Here's the drawing with two shaded views (mm, measured from the low corner). I have some questions. Coordinates: 2 decimals unless noted, no trailing zeros. Order: outer loops, then holes, each group sorted by start corner. A loop starts at its lowest first (then second) coordinate and runs counter-clockwise, first axis right, second up. Notation, with made-up numbers: (62, -34.75) -> (66, -34.75) arc R36 ccw to (66, 3.25) -> close; hole circle Ø6 at (-31, 24). An arc over 180 degrees is marked (long way). Answer in a Markdown table with one row per item. Add a question column.
1. If I drill on line 1 along X through (y, z) = (2.9, 30); line 2 along Y through (x, z) = (7.5, 27); line 3 along Z through (x, y) = (18, 4.2), over which ranges is the centre line in solid material (lowest first)? Write a range as [from, to].
2. Imagine slicing it at A-A on x = 16. Write out the boundary of the cut face in (y, z).
3. Imagine slicing it at D-D on x = 50.5. Write out the boundary of the cut face in (y, z).
4. Imagine slicing it at C-C on y = 2.7. Write out the boundary of the cut face in (x, z), plus the area to 3 significant figures.
5. Imagine slicing it at B-B on z = 25. Write out the boundary of the cut face in (x, y), plus the area to 3 significant figures.
6. Will these pins go through, and if not, where does the flat tip stop? pin 1 (1.5 mm diameter, centred on x = 22.5, y = 3, fed in from +Z); pin 2 (1.5 mm diameter, centred on y = 3, z = 16.5, fed in from +X).
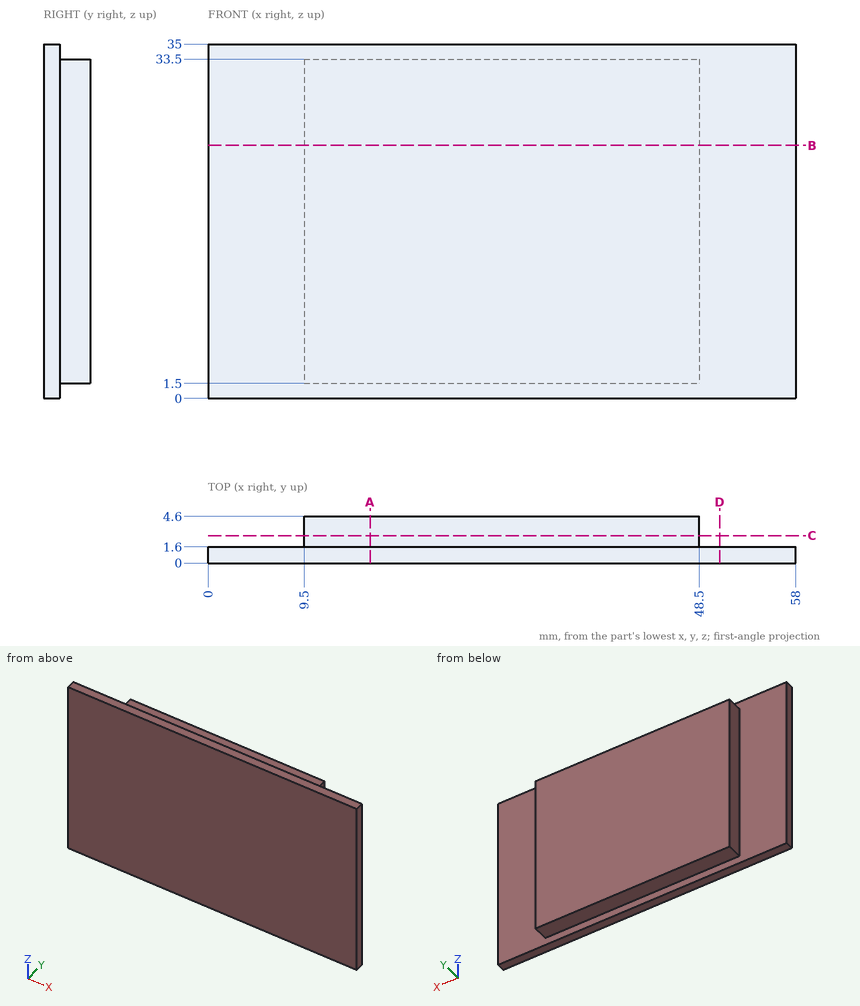
Answers follow:
| question | item | result |
|---|---|---|
| 1 | line 1 | x = [9.5, 48.5] |
| 1 | line 2 | y = [0, 1.6] |
| 1 | line 3 | z = [1.5, 33.5] |
| 2 | outline | (0, 0) -> (1.6, 0) -> (1.6, 1.5) -> (4.6, 1.5) -> (4.6, 33.5) -> (1.6, 33.5) -> (1.6, 35) -> (0, 35) -> close |
| 3 | outline | (0, 0) -> (1.6, 0) -> (1.6, 35) -> (0, 35) -> close |
| 4 | outline | (9.5, 1.5) -> (48.5, 1.5) -> (48.5, 33.5) -> (9.5, 33.5) -> close |
| 4 | area | 1,250 mm² |
| 5 | outline | (0, 0) -> (58, 0) -> (58, 1.6) -> (48.5, 1.6) -> (48.5, 4.6) -> (9.5, 4.6) -> (9.5, 1.6) -> (0, 1.6) -> close |
| 5 | area | 210 mm² |
| 6 | pin 1 | stops at z = 33.5 |
| 6 | pin 2 | stops at x = 48.5 |
